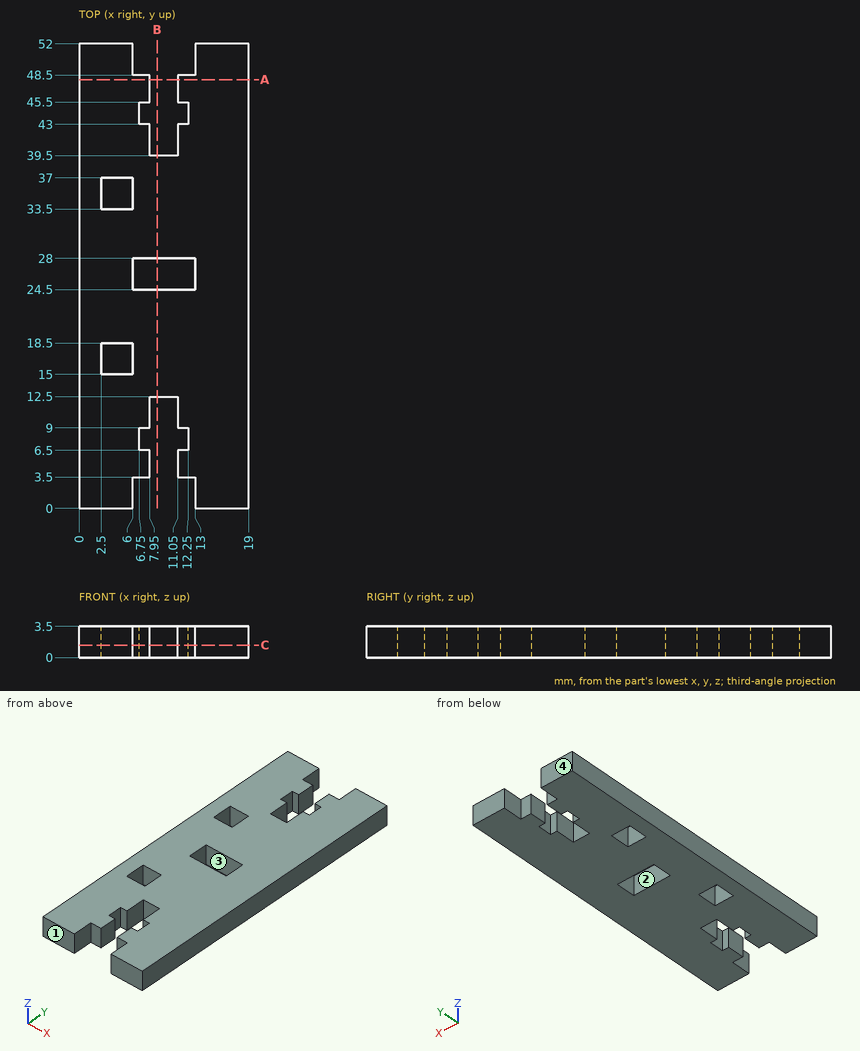
Check sheet for the drawn part. Datum: minimum x, y, z corner. Units: mm. A direction names the side the tool comes from. Coordinates: 2 decimals unless noted, no trailing zeros. Loops run counter-clockwise (first coordinate to the right, second up) from the corner with the lowest first, then second, coordinate; pieces in that order, holes last. Notation, with made-up numbers: (78.25, -36) -> (121.25, -36) arc R22 cw to (121.25, 3) -> close; hole circle Ø7 at (-17.5, 61.25). An arc over 180 degrees is marked (long way). Answer in a Markdown table with one row per item.
1) Section check B-B (x = 8.75). Record the cut outline in (y, z).
The answers:
| item | result |
|---|---|
| outline | (12.5, 0) -> (24.5, 0) -> (24.5, 3.5) -> (12.5, 3.5) -> close; (28, 0) -> (39.5, 0) -> (39.5, 3.5) -> (28, 3.5) -> close |
2) Depth check by flat-ended pin: P1, Ø0.9, axis at x = 9, z = 1.5, coming from the -Y side; P2, Ø0.6, axis at x = 12, z = 2.5, coming from the +Y side; P3, Ø1, axis at x = 11, z = 2, coming from the -Y side. Enter the tip coordinate at first touch or a pass-through.
The answers:
| item | result |
|---|---|
| P1 | stops at y = 12.5 |
| P2 | stops at y = 48.5 |
| P3 | stops at y = 3.5 |
3) Section check A-A (y = 48). Record the cut outline in (x, z), and give its area (4 significant figures).
The answers:
| item | result |
|---|---|
| outline | (0, 0) -> (7.95, 0) -> (7.95, 3.5) -> (0, 3.5) -> close; (11.05, 0) -> (19, 0) -> (19, 3.5) -> (11.05, 3.5) -> close |
| area | 55.65 mm2 |
4) Section check C-C (z = 1.4). Give the number of separate pieces and of enclosed holes in the cut face, and give its area (3 significant figures).
The answers:
| item | result |
|---|---|
| separate pieces | 1 |
| enclosed holes | 3 |
| area | 822 mm2 |
5) Scan lines: line 1 along Y through (x, z) = (3.5, 1.75); line 2 along X through (y, z) = (27, 3); line 3 along X through (y, z) = (6, 0.4). Record each from-to range of solid material in increasing order. Write a range as from..to.
The answers:
| item | result |
|---|---|
| line 1 | y = 0..15, 18.5..33.5, 37..52 |
| line 2 | x = 0..6, 13..19 |
| line 3 | x = 0..7.95, 11.05..19 |
6) Access from +Z, -Z, +X, -X, +Y, -Y to the whole of each face (thin tool, end or side, straight path). Record for the marked faces 3 and 4.
The answers:
| item | result |
|---|---|
| face 3 | +Z, -Z |
| face 4 | +Z, -Z, +X, -X, +Y |
7) Draft check along X on the marked faces 1 and 2. Enter one of: released by +X, released by -X, zero draft, split by the parting line, or undercut.
The answers:
| item | result |
|---|---|
| face 1 | zero draft |
| face 2 | undercut |
